Could you check a few things on this drawing? It's one solid part, dimensions in mm from its lowest x, y, z. A direction names the side the tool comes from. Round coordinates to 2 decimals unless told otherwise and drop trailing zeros. Loops run counter-clockwise (first coordinate to the right, second up) from the corner with the lowest first, then second, coordinate; pieces in that order, holes last. Notation, with made-up numbers: M 57,2 L 75,2 A5 ccw 75,10 Z; hole C 76,10 d4. An arc over 180 degrees is marked long. Use a Markdown table: item, result. Add a question column.
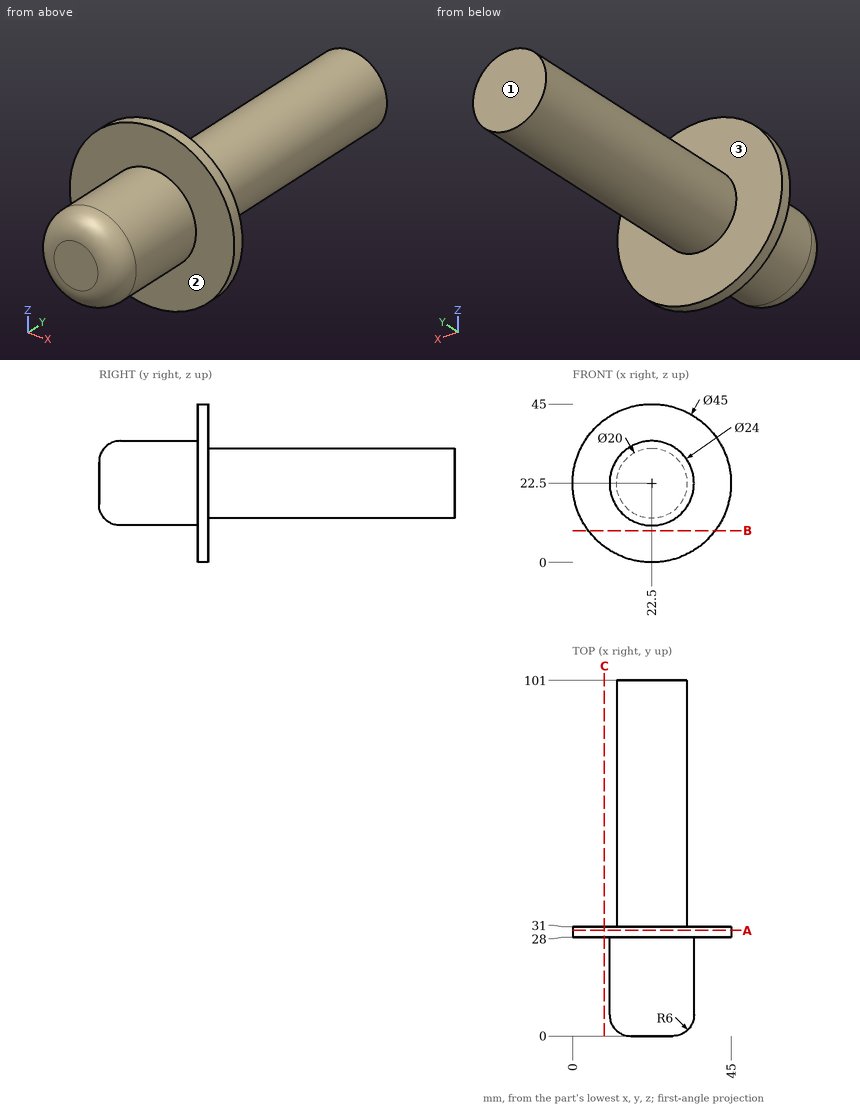
(1) I'm going to push flat-ended pins straight in: pin 1 (5 mm diameter, centred on y = 18.5, z = 13.5, fed in from +X); pin 2 (1 mm diameter, centred on x = 11.5, y = 19.5, fed in from -Z); pin 3 (2 mm diameter, centred on x = 28.5, y = 53, fed in from -Z). Where does each tip first touch, or does it pass through?
(2) Suppose I cut it at B-B on z = 9. List the corners of the cut face in (x, y) for me, and give its area (3 significant figures).
(3) Suppose I cut it at C-C on x = 9. List the corners of the cut face in (y, z) for me.
(4) Suppose I cut it at A-A on y = 30. List the corners of the cut face in (x, z) for me.
(5) If I drill on probe 1 along Y at (x, z) = (18, 41); probe 2 along Z at (x, y) = (14.5, 46.5); probe 3 along Y at (x, z) = (28, 19.5), over which ranges is the centre line in solid material (lowest first)? Write a range as [from, to].
(6) On a 3-axis mill with a long thin cutter (end or side, diameter ignored), from which of +Z, -Z, +X, -X, +Y, -Y can I reach the whole of each face in a straight line? I mean the marked faces 1, 2 and 3. Say none if no direction works.
Results below:
| question | item | result |
|---|---|---|
| 1 | pin 1 | stops at x = 32.59 |
| 1 | pin 2 | stops at z = 16.69 |
| 1 | pin 3 | stops at z = 13.84 |
| 2 | outline | M 4.5,28 L 40.5,28 L 40.5,31 L 4.5,31 Z |
| 2 | area | 108 mm² |
| 3 | outline | M 28,4.5 L 31,4.5 L 31,40.5 L 28,40.5 Z |
| 4 | outline | C 22.5,22.5 d45 |
| 5 | probe 1 | y = [28, 31] |
| 5 | probe 2 | z = [16.5, 28.5] |
| 5 | probe 3 | y = [0.01, 101] |
| 6 | face 1 | +Z, -Z, +X, -X, +Y |
| 6 | face 2 | -Y |
| 6 | face 3 | +Y |
